Check sheet for the drawn part. Datum: minimum x, y, z corner. Units: mm. A direction names the side the tool comes from. Coordinates: 2 decimals unless noted, no trailing zeros. Write each loop counter-clockwise with the first axis right and the second up, starting at its lowest first coordinate (ties: lowest second). Pieces come first, ordered by that corner, then holes. Notation, with made-up numbers: M -15,-31 L -2,-31 A15 cw -2,-19 Z; hole C 64,39 d8. An arc over 180 degrees is marked long. Answer in a Markdown table with one row per item.
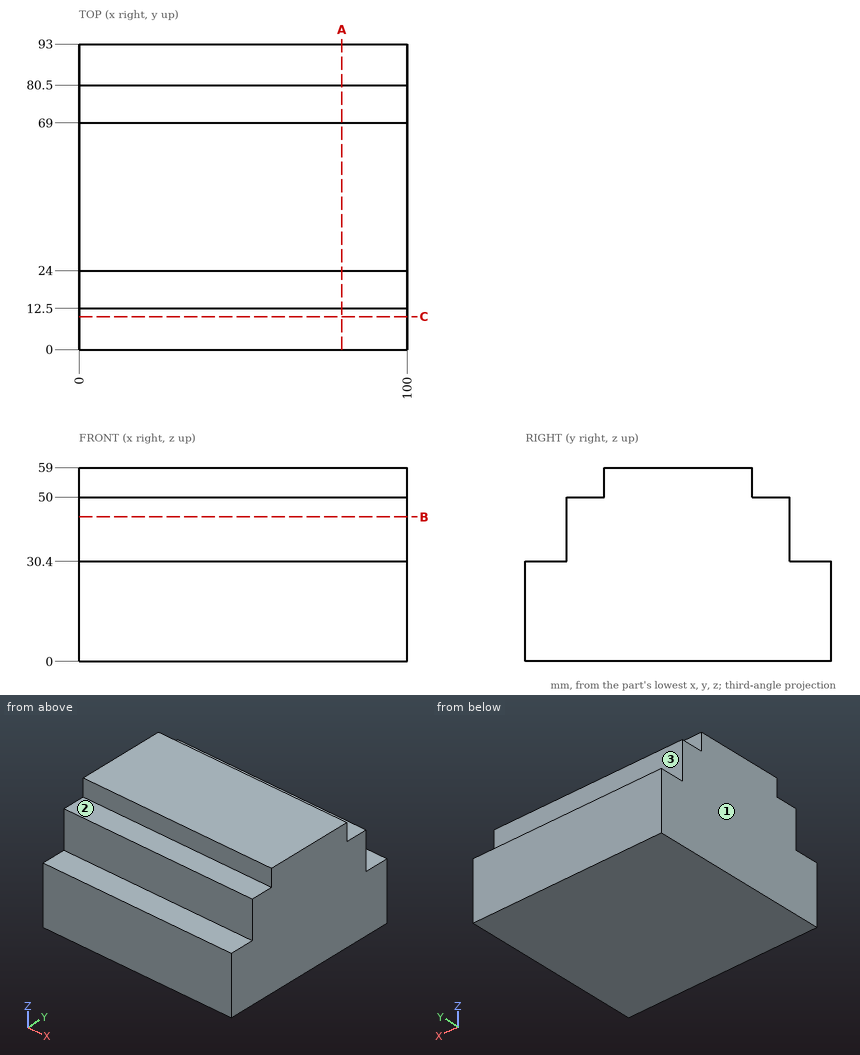
1) Sectioned sample at A-A (x = 80). Record the cut outline in (y, z), then the cut area to 4 significant figures.
Response values:
| item | result |
|---|---|
| outline | M 0,0 L 93,0 L 93,30.4 L 80.5,30.4 L 80.5,50 L 69,50 L 69,59 L 24,59 L 24,50 L 12.5,50 L 12.5,30.4 L 0,30.4 Z |
| area | 4,565 mm² |
2) Thickness scan on L1, parallel to Y at x = 77.5, z = 55; L2, parallel to Y at x = 19, z = 44.5; L3, parallel to Z at x = 68.5, y = 19.5. Record the ranges inside material, lowest first. Write a range as [from, to].
Response values:
| item | result |
|---|---|
| L1 | y = [24, 69] |
| L2 | y = [12.5, 80.5] |
| L3 | z = [0, 50] |
3) Tool access check on the marked faces 1, 2 and 3. Record the directions out of +Z, -Z, +X, -X, +Y, -Y that give a thin tool (end or side, any length) a straight path to the whole face; none if there is none.
Response values:
| item | result |
|---|---|
| face 1 | +Z, -Z, -X, +Y, -Y |
| face 2 | +Z, +X, -X, -Y |
| face 3 | +Z, +X, -X, +Y |
4) Sectioned sample at B-B (z = 44). Record the cut outline in (x, y).
Response values:
| item | result |
|---|---|
| outline | M 0,12.5 L 100,12.5 L 100,80.5 L 0,80.5 Z |
5) Sectioned sample at C-C (y = 10). Record the cut outline in (x, z), then the cut area to 3 significant figures.
Response values:
| item | result |
|---|---|
| outline | M 0,0 L 100,0 L 100,30.4 L 0,30.4 Z |
| area | 3,040 mm² |
6) Depth check by flat-ended pin: pin 1 (21.5 mm diameter, centred on x = 71, z = 41.5, fed in from +Y); pin 2 (2.5 mm diameter, centred on x = 63, z = 55, fed in from -Y); pin 3 (14 mm diameter, centred on x = 45.5, y = 84, fed in from +Z). Enter the tip coordinate at first touch or a pass-through.
Response values:
| item | result |
|---|---|
| pin 1 | stops at y = 80.5 |
| pin 2 | stops at y = 24 |
| pin 3 | stops at z = 50 |
